The model under review builds one solid part; all positions refer to its coordinate system, in mm. A direction names the side the tool comes from. Give positions to 0.01 mm unless a question says otherwise; leave off trailing zeros. Loops run counter-clockwise (first coordinate to the right, second up) from the corner with the lowest first, then second, coordinate; pieces in that order, holes last. Notation, with made-up numbers: (-26.5, -9.75) -> (-11.5, -9.75) arc R24 ccw to (-11.5, 24.25) -> close; hole circle Ø1 at (77.5, -31.5). An arc over 180 degrees is marked (long way). Write each question's results on one line, items separated by ' | '. Start each with the question number.
Q1. Insertion check: pin 1 Ø3 at (x, y) = (-82.5, 8.5) entering from -Z; pin 2 Ø3 at (x, z) = (-78, 15.5) entering from +Y; pin 3 Ø6 at (x, z) = (-80, 9) entering from -Y. Each pin has a flat end and moves straight along its axis. Give the tip position at first contact, or say it passes through.
Q2. Mouldability with a two-part tool opening along Z and no side actions: class faces 1 (the face through (-83, 113, 25.4)), 2 (the face through (-88.7, 110, 13)), 3 (the face through (-85.7, 212.9, 12.6)), 4 (the face through (-86, 191, 9.7)) as released by +Z, released by -Z, zero draft, split by the parting line, or undercut.
Q3. Machinability: for faces 5 (the face through (-84.548, 11.28, 19.138)), 6 (the face through (-82.75, 190, 16)), 7 (the face through (-86, 190, 15.7)), which of the approach directions +Z, -Z, +X, -X, +Y, -Y give a long, thin tool a straight path to every point of the face, cutting with its end or side? Answer none if there is none.
Q4. We need section C-C (z = 19.05). Write out the cut boundary in (x, y).
Q5. We need section B-B (x = -86.75). Write out the cut boundary in (y, z), plus the area to 3 significant figures.
Q6. Wall thickness on L1, parallel to Z at x = -82.55, y = 10.25; L2, parallel to Y at x = -87.5, z = 3.75; L3, parallel to Y at x = -78.25, z = 16.75: over which ranges is each line inside the solid? List them lowest first. Write a range as [from, to].
Q7. We need section A-A (y = 188). Write out the cut boundary in (x, z), plus the area to 3 significant figures.
from build123d import *

# Parameters (mm, degrees)
SKETCH009_W     = 12.3
SKETCH009_H     = 209.55
PAD002_DEPTH    = 25.4
SKETCH010_W     = 12.3
SKETCH010_H     = 6.35
POCKET007_DEPTH = 12.7
SKETCH011_R     = 2
POCKET008_DEPTH = 10
SKETCH012_W     = 6.35
SKETCH012_H     = 50.8
POCKET009_DEPTH = 25.401
POCKET010_DEPTH = 5.951


with BuildPart() as part:
    # Sketch009 → Pad002 (new body)
    with BuildSketch(Plane.XY):
        with Locations((-82.55, 111.125)):
            Rectangle(SKETCH009_W, SKETCH009_H)
    extrude(amount=PAD002_DEPTH)

    # Sketch010 (on Face5 of Pad002) → Pocket007 (cut)
    with BuildSketch(Plane(origin=(0, 0, 0), x_dir=(1, 0, 0), z_dir=(0, 0, -1))):
        with Locations((-82.55, -9.525)):
            Rectangle(SKETCH010_W, SKETCH010_H)
    extrude(amount=-POCKET007_DEPTH, mode=Mode.SUBTRACT)

    # Sketch011 (on Face1 of Pocket007) → Pocket008 (cut)
    with BuildSketch(Plane.XZ.offset(-6.35)):
        with Locations((-82.55, 19.05)):
            Circle(SKETCH011_R)
    extrude(amount=-POCKET008_DEPTH, mode=Mode.SUBTRACT)

    # Sketch012 (on Face5 of Pocket008) → Pocket009 (cut, through all)
    with BuildSketch(Plane.XY.offset(25.4)):
        with Locations((-79.575, 190.5)):
            Rectangle(SKETCH012_W, SKETCH012_H)
    extrude(amount=-POCKET009_DEPTH, mode=Mode.SUBTRACT)

    # Sketch013 (on Face11 of Pocket009) → Pocket010 (cut, through all)
    with BuildSketch(Plane.YZ.offset(-82.75)):
        with BuildLine():
            Line((171.1, 15.7), (209.9, 15.7))
            ThreePointArc((209.9, 9.7), (212.9, 12.7), (209.9, 15.7))
            Line((209.9, 9.7), (171.1, 9.7))
            ThreePointArc((171.1, 15.7), (168.1, 12.7), (171.1, 9.7))
        make_face()
    extrude(amount=-POCKET010_DEPTH, mode=Mode.SUBTRACT)


solid = part.part
Output:
1) pin 1: z = 12.7 | pin 2: y = 165.1 | pin 3: y = 12.7
2) face 1: released by +Z | face 2: zero draft | face 3: undercut | face 4: undercut
3) face 5: -Y | face 6: +Z, -Z, +X, +Y | face 7: +X, -X
4) outline: (-88.7, 6.35) -> (-84.55, 6.35) -> (-84.55, 16.35) -> (-80.55, 16.35) -> (-80.55, 6.35) -> (-76.4, 6.35) -> (-76.4, 165.1) -> (-82.75, 165.1) -> (-82.75, 215.9) -> (-88.7, 215.9) -> close
5) outline: (6.35, 12.7) -> (12.7, 12.7) -> (12.7, 0) -> (215.9, 0) -> (215.9, 25.4) -> (6.35, 25.4) -> close; hole (171.1, 9.7) -> (209.9, 9.7) arc R3 ccw to (209.9, 15.7) -> (171.1, 15.7) arc R3 ccw to start | area: 4,980 mm2
6) L1: [12.7, 17.05], [21.05, 25.4] | L2: [12.7, 215.9] | L3: [6.35, 165.1]
7) outline: (-88.7, 0) -> (-82.75, 0) -> (-82.75, 9.7) -> (-88.7, 9.7) -> close; (-88.7, 15.7) -> (-82.75, 15.7) -> (-82.75, 25.4) -> (-88.7, 25.4) -> close | area: 115 mm2
